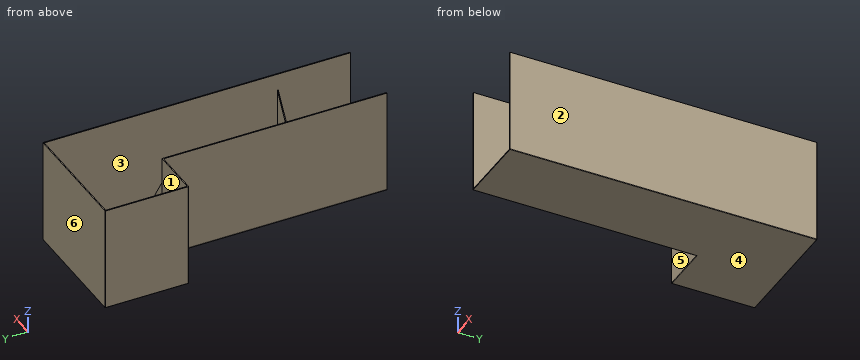
from build123d import *

# Parameters (mm, degrees)
F1_DEPTH  = 426
F3_DEPTH  = 4
F4_R      = 2
F7_DEPTH  = 4
F10_DEPTH = 4


# Not quite as in the source:
# - a feature names something its author has since deleted; it is built from what else it names


with BuildPart() as f1:
    # F0 (on Top) → F1 (new body)
    with BuildSketch(Plane.XY):
        Polygon((495, 0), (0, 0), (0, -343), (200, -343), (200, -1261), (204, -1261), (204, -339), (4, -339), (4, -4), (491, -4), (491, -1261), (495, -1261), align=None)
    extrude(amount=F1_DEPTH)

    # F2 (on Top) → F3 (join)
    with BuildSketch(Plane.XY):
        Polygon((0, -343), (200, -343), (199.9874711037, -1261), (495, -1261), (495, 0), (0, 0), align=None)
    extrude(amount=-F3_DEPTH)

    # F4
    f4_edges = [f1.edges().sort_by_distance(p)[0] for p in [
        (100, -343, -4),
        (0, -171.5, -4),
        (247.5, 0, -4),
        (0, -343, 211),
        (0, 0, 211),
        (495, 0, 211),
        (199.993736, -802, -4),
        (495, -630.5, -4),
    ]]
    fillet(f4_edges, radius=F4_R)

    # F6 (on offset) → F7 (join)
    with BuildSketch(Plane.XZ.offset(961)):
        Polygon((269, 0), (491, 0), (491, 355), align=None)
    extrude(amount=F7_DEPTH)

    # F9 (on offset) → F10 (join)
    with BuildSketch(Plane.XZ.offset(361)):
        Polygon((204, 355), (204, 0), (426, 0), align=None)
    extrude(amount=F10_DEPTH)


solid = f1.part
CAD build for the part. Positions are in the model's coordinates, mm. Face numbers are marked on the shaded views. A direction names the side the tool comes from. Round coordinates to 2 decimals unless told otherwise and drop trailing zeros. Loops run counter-clockwise (first coordinate to the right, second up) from the corner with the lowest first, then second, coordinate; pieces in that order, holes last. Notation, with made-up numbers: M 10.25,-7 L 35.25,-7 A14 ccw 35.25,-3 Z; hole C 37,87.5 d3. An arc over 180 degrees is marked long. One line per question, with ' | ' between items. Start each with the question number.
Item 1: Wall check: line 1 (Y direction, x = 261, z = 258); line 2 (X direction, y = -941.5, z = 158); line 3 (Y direction, x = 350.5, z = 20.5). Give the ranges that are in metal, low to high.
Item 2: Cut at C-C, the plane z = 115. Write the cut outline in (x, y), plus the area to 3 significant figures.
Item 3: Two-plate mould, pull along X, no slides. Class the marked faces 1, 2, 3 and 4: pulls with the +X half, pulls with the -X half, needs draft (parallel to the pull), parting line crosses it, or undercut.
Item 4: Which spindle directions (+Z, -Z, +X, -X, +Y, -Y) get a long thin tool onto all of the face, cutting with end or side? Do the marked faces 5 and 6. Say none if no direction does.
Item 5: Cut at A-A, the plane x = 80.5. Write the cut outline in (y, z).
Item 6: Cut at D-D, the plane x = 252.5. Write the cut outline in (y, z).
Item 7: Pin check, flat tips, straight feed: pin 1 Ø1.5 at (x, z) = (312.5, 250) entering from -Y; pin 2 Ø1.6 at (y, z) = (-704, -0.5) entering from -X; pin 3 Ø4 at (x, z) = (144.5, 44.5) entering from -Y. Stop position of each tip, or through.
Item 8: Cut at B-B, the plane y = -165. Write the cut outline in (x, z), plus the area to 3 significant figures.
Responses:
1) line 1: y = -365 to -361, -4 to 0 | line 2: x = 200 to 204, 491 to 495 | line 3: y = -965 to -961, -365 to -361, -4 to 0
2) outline: M 0,-341 A2 ccw 2,-343 L 200,-343 L 200,-1261 L 204,-1261 L 204,-365 L 354.08,-365 L 354.08,-361 L 204,-361 L 204,-339 L 4,-339 L 4,-4 L 491,-4 L 491,-961 L 340.92,-961 L 340.92,-965 L 491,-965 L 491,-1261 L 495,-1261 L 495,-2 A2 ccw 493,0 L 2,0 A2 ccw 0,-2 Z | area: 14,000 mm²
3) face 1: undercut | face 2: pulls with the +X half | face 3: undercut | face 4: needs draft
4) face 5: +Z, -Z, -X, -Y | face 6: +Z, -Z, +X, -X, +Y
5) outline: M -343,-2 A2 ccw -341,-4 L -2,-4 A2 ccw 0,-2 L 0,426 L -4,426 L -4,0 L -339,0 L -339,426 L -343,426 Z
6) outline: M -1261,-4 L -2,-4 A2 ccw 0,-2 L 0,426 L -4,426 L -4,0 L -361,0 L -361,277.44 L -365,277.44 L -365,0 L -1261,0 Z
7) pin 1: stops at y = -4 | pin 2: stops at x = 200 | pin 3: stops at y = -343
8) outline: M 0,-2 A2 ccw 2,-4 L 493,-4 A2 ccw 495,-2 L 495,426 L 491,426 L 491,0 L 4,0 L 4,426 L 0,426 Z | area: 5,390 mm²
